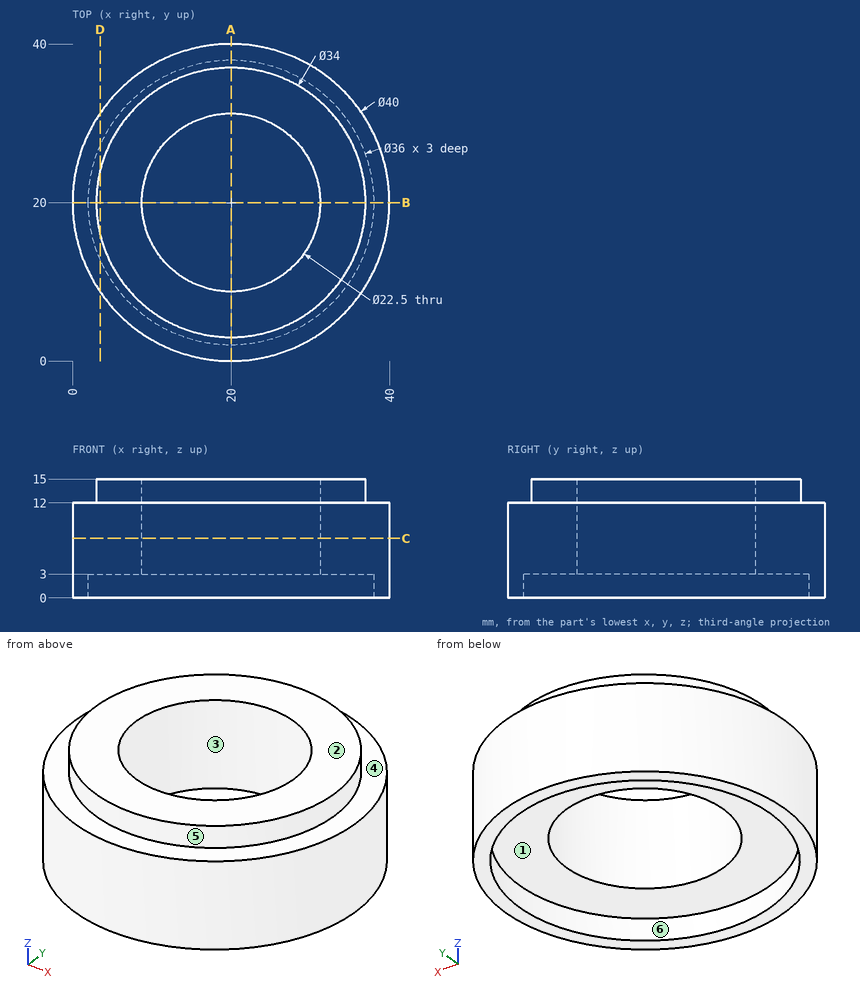
Geometry check sheet. Reference: drawing and pictorial views, mm from the part's lowest x, y, z. A direction names the side the tool comes from. Round coordinates to 2 decimals unless told otherwise and drop trailing zeros. Order: outer loops, then holes, each group sorted by start corner. A loop starts at its lowest first (then second) coordinate and runs counter-clockwise, first axis right, second up.
Q1. Scan lines: L1, parallel to Y at x = 20, z = 1; L2, parallel to Y at x = 20, z = 7.25; L3, parallel to Z at x = 16.5, y = 7.5. Record each from-to range of solid material in increasing order.
Filled sheet:
L1: y = 0 to 2, 38 to 40
L2: y = 0 to 8.75, 31.25 to 40
L3: z = 3 to 15
Q2. Cross-section at A-A, the plane x = 20. Enter the section's corners in (y, z).
Filled sheet:
outline: (0, 0) - (2, 0) - (2, 3) - (8.75, 3) - (8.75, 15) - (3, 15) - (3, 12) - (0, 12) - close; (31.25, 3) - (38, 3) - (38, 0) - (40, 0) - (40, 12) - (37, 12) - (37, 15) - (31.25, 15) - close
Q3. Cross-section at C-C, the plane z = 7.5. Enter the section's corners in (x, y), plus the area to 3 significant figures.
Filled sheet:
outline: circle Ø40 at (20, 20); hole circle Ø22.5 at (20, 20)
area: 859 mm2
Q4. Cross-section at D-D, the plane x = 3.5. Enter the section's corners in (y, z), plus the area to 3 significant figures.
Filled sheet:
outline: (8.7, 0) - (12.81, 0) - (12.81, 3) - (27.19, 3) - (27.19, 0) - (31.3, 0) - (31.3, 12) - (24.09, 12) - (24.09, 15) - (15.91, 15) - (15.91, 12) - (8.7, 12) - close
area: 253 mm2
Q5. Depth check by flat-ended pin: P1, Ø5, axis at x = 35, z = 12, coming from the +Y side; P2, Ø3, axis at x = 6.5, z = 11, coming from the +Y side; P3, Ø3, axis at x = 35, z = 8.5, coming from the -Y side; P4, Ø1, axis at x = 28.5, y = 26.5, coming from the -Z side. Enter the tip coordinate at first touch or a pass-through.
Filled sheet:
P1: stops at y = 35.61
P2: stops at y = 36
P3: stops at y = 5.24
P4: passes through
Q6. Draft check along Y on the marked faces 3, 4, 5 and 6. Enter one of: pulls with the +Y half, pulls with the -Y half, needs draft (parallel to the pull), parting line crosses it, or undercut.
Filled sheet:
face 3: undercut
face 4: needs draft
face 5: parting line crosses it
face 6: undercut
Q7. Set-up check for the marked faces 1 and 2: record each of +Z, -Z, +X, -X, +Y, -Y from which the full face is reachable in a straight line by a thin tool's end or side.
Filled sheet:
face 1: -Z
face 2: +Z, +X, -X, +Y, -Y
